The drawing under review shows one solid part. Ordinate dimensions are in mm from its lowest x, y, z. Coordinates: 2 decimals unless noted, no trailing zeros. Write each loop counter-clockwise with the first axis right and the second up, starting at its lowest first coordinate (ties: lowest second). Pieces come first, ordered by that corner, then holes. Notation, with made-up numbers: (0, -2) - (28, -2) arc R23 cw to (28, 19) - close; hole circle Ø6 at (12, -13). An arc over 180 degrees is marked (long way). Answer as CSV lines item,"result". Start each with the question number.
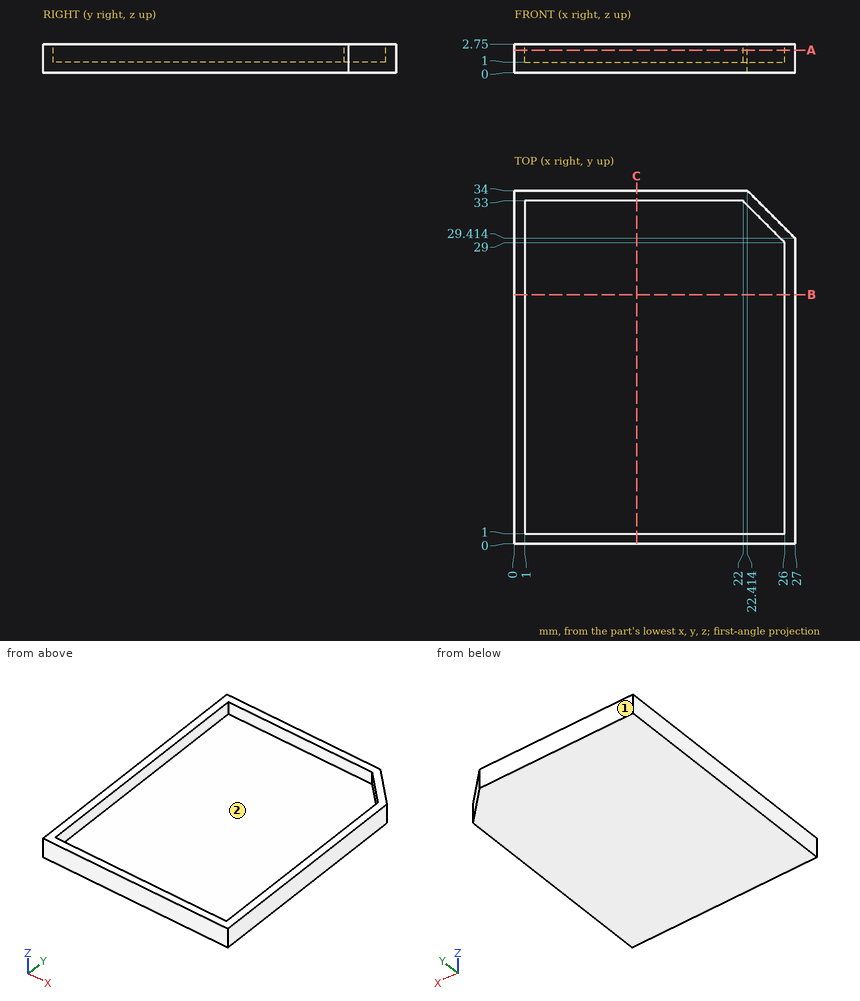
(1) Add section A-A on z = 2.15. Give the boundary of the cut face in (x, y).
(2) For pin 1 (7.5 mm diameter, centred on x = 16, y = 24.5, fed in from +Z), flat-tipped, find the tip position at first contact; note if it passes through.
(3) Add section C-C on x = 11.75. Give the boundary of the cut face in (y, z).
(4) Add section B-B on y = 24. Give the boundary of the cut face in (x, z).
(5) Wall thickness on line 1 (X direction, y = 5, z = 2.2); line 2 (Y direction, x = 19.5, z = 1.6); line 3 (Z direction, x = 14, y = 28): over which ranges is each line inside the solid? List them lowest first.
(6) The part is to be moulded in two halves that separate along X. For the marked faces 1 and 2, say which applies: released by +X, released by -X, zero draft, split by the parting line, or undercut.
Reported:
1,outline,"(0, 0) - (27, 0) - (27, 29.41) - (22.41, 34) - (0, 34) - close; hole (1, 1) - (26, 1) - (26, 29) - (22, 33) - (1, 33) - close"
2,pin 1,"z = 1"
3,outline,"(0, 0) - (34, 0) - (34, 2.75) - (33, 2.75) - (33, 1) - (1, 1) - (1, 2.75) - (0, 2.75) - close"
4,outline,"(0, 0) - (27, 0) - (27, 2.75) - (26, 2.75) - (26, 1) - (1, 1) - (1, 2.75) - (0, 2.75) - close"
5,line 1,"0 to 1, 26 to 27"
5,line 2,"0 to 1, 33 to 34"
5,line 3,"0 to 1"
6,face 1,"zero draft"
6,face 2,"undercut"
